Could you check a few things on this model? Use its own coordinates, in mm. Round coordinates to 2 decimals unless told otherwise and drop trailing zeros. Order: outer loops, then holes, each group sorted by start corner. A loop starts at its lowest first (then second) coordinate and runs counter-clockwise, first axis right, second up. Notation, with made-up numbers: (22.5, 32) - (37.5, 32) arc R29 cw to (37.5, 55) - close; hole circle Ø10 at (13.25, -19.75). An arc over 180 degrees is marked (long way). Use one line per item in the form item = value.
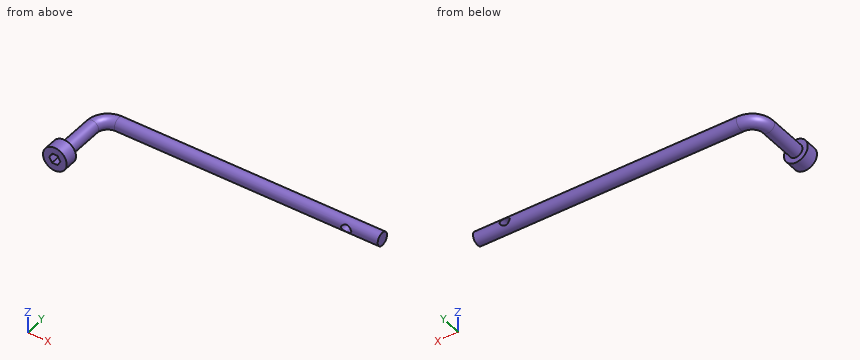
Autodesk Inventor part; units mm, degrees
ref_plane "YZ Plane" through (0, 0, 0) normal (1, 0, 0) x (0, 1, 0)
ref_plane "XZ Plane" through (0, 0, 0) normal (0, 1, 0) x (-1, 0, 0)
ref_plane "XY Plane" through (0, 0, 0) normal (0, 0, 1) x (1, 0, 0)
sketch "Sketch1" plane through (0, 0, 0) normal (0, 1, 0) x (-1, 0, 0)
  arc A0 (-450, 0) -> (-430, 0) centre (-440, 3.6429) ccw
  arc A1 (-430, 0) -> (-450, 0) centre (-440, -3.6429) ccw
sketch "Sketch2" plane through (0, 0, 0) normal (1, 0, 0) x (0, 1, 0)
  circle A0 centre (0, 0) radius 12.5
  dimension "d8" = 25
extrude "Extrusion1" add sketch "Sketch2" along normal blind 500
extrude "Extrusion2" cut sketch "Sketch1" along normal mid plane 25
sketch "Sketch3" plane through (0, 0, 0) normal (0, 0, 1) x (1, 0, 0)
  line L0 (0, -12.5) -> (0, 12.5)
  line L1 (0, -30) -> (-42.5, -30) construction
  line L2 (0, -30) -> (0, 12.5) construction
  line L3 (-17.5, -30) -> (-17.5, -105)
  line L4 (-17.5, -105) -> (-7.5, -105)
  line L5 (-7.5, -105) -> (-7.5, -130)
  line L6 (-7.5, -130) -> (-30, -130)
  line L7 (-30, -130) -> (-30, -30)
  line L8 (-17.5, -30) -> (-30, -30)
  point P0 (0, 0)
  point P1 (0, 0)
  dimension "d13" = 90
  dimension "d14" = 30
  dimension "d15" = 75
  dimension "d16" = 10
  dimension "d17" = 25
  dimension "d18" = 22.5
revolve "Revolution1" add sketch "Sketch3" angle 360 about axis through (-30, -130, 0) along (0, 1, 0)
sketch "Sketch5" plane through (0, 0, 0) normal (-1, 0, 0) x (0, 0, 1)
  circle A0 centre (0, 0) radius 12.5
  line L0 (12.5, -30) -> (-12.5, -30)
  line L1 (12.5, -30) -> (-12.5, -30)
revolve "Revolution2" add sketch "Sketch5" angle 90 about axis through (0, -30, 12.5) along (0, 0, 1)
sketch "Sketch6" plane through (-30, -130, 0) normal (0, -1, 0) x (1, 0, 0)
  line L0 (-10.5, -0.0258) -> (-5.25, 9.0675)
  line L1 (-5.25, 9.0675) -> (5.25, 9.0675)
  line L2 (5.25, 9.0675) -> (10.5, -0.0258)
  line L3 (10.5, -0.0258) -> (5.25, -9.119)
  line L4 (5.25, -9.119) -> (-5.25, -9.119)
  line L5 (-5.25, -9.119) -> (-10.5, -0.0258)
  circle A0 centre (0, 0) radius 22.5
  point P0 (30, 0)
  point P1 (0, 9.0675)
  dimension "d24" = 120
  dimension "d25" = 21
  dimension "d26" = 120
  dimension "d27" = 120
  dimension "d28" = 0
  dimension "d29" = 120
  dimension "d30" = 0
  dimension "d31" = 10.5
  dimension "d32" = 10.5
extrude "Extrusion3" cut sketch "Sketch6" against normal blind 20 contours L0 L1 L2 L3 L4 L5
properties part number "Chave" material "Steel ASTM A36"
Item 1: Imagine slicing it at B-B on y = -53.5. Please give me the cut outline in (x, z), plus the area to 3 significant figures.
Found:
outline = circle Ø25 at (-30, 0)
area = 491 mm2
Item 2: Imagine slicing it at C-C on x = 438.5. Please give me the cut outline in (y, z), plus the area to 3 significant figures.
Found:
outline = (-10.43, -6.89) arc R12.5 ccw to (10.43, -6.89) - close; (-10.43, 6.89) - (10.43, 6.89) arc R12.5 ccw to start
area = 165 mm2
Item 3: Imagine slicing it at A-A on x = 39.5. Please give me the cut outline in (y, z).
Found:
outline = circle Ø25 at (0, 0)
Item 4: Will these pins go through, and if not, where does the flat tip stop? P1, Ø20, axis at x = -34.5, z = 4, coming from the -Y side; P2, Ø5, axis at x = -32, y = -115.5, coming from the -Z side; P3, Ø12, axis at y = -6, z = -15.5, coming from the -X side; P4, Ø5, axis at x = 92, z = 3.5, coming from the -Y side.
Found:
P1 = -130
P2 = -22.5
P3 = -30.65
P4 = -12.46
Item 5: I need wall thicknesses on L1, parallel to X at y = -109.5, z = 0; L2, parallel to X at y = -112.5, z = -7; L3, parallel to X at y = -28, z = -0.5. Which ranges of each line are inside material? Lowest first, please.
Found:
L1 = -52.5 to -7.5
L2 = -51.38 to -36.47, -23.53 to -8.62
L3 = -42.44 to -17.4
